from build123d import *

# Parameters (mm, degrees)
ESQUISSE1_R        = 3.9751
BOSS_EXTRU_1_DEPTH = 38.1
BOSS_EXTRU_2_DEPTH = 6.35


with BuildPart() as part:
    # Esquisse1 → Boss.-Extru.1 (new body)
    with BuildSketch(Plane.XY):
        Circle(ESQUISSE1_R)
    extrude(amount=-BOSS_EXTRU_1_DEPTH)

    # Esquisse2 → Boss.-Extru.2 (add)
    with BuildSketch(Plane.XY):
        Polygon((8.248891971, 0), (4.124445986, 7.14375), (-4.124445986, 7.14375), (-8.248891971, 0), (-4.124445986, -7.14375), (4.124445986, -7.14375), align=None)
    extrude(amount=BOSS_EXTRU_2_DEPTH)


solid = part.part
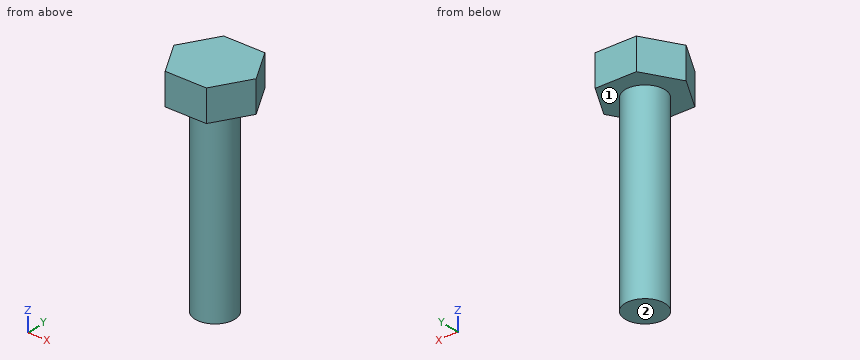
CAD build for the part. Positions are in the model's coordinates, mm. Face numbers are marked on the shaded views. A direction names the side the tool comes from. Coordinates: 2 decimals unless noted, no trailing zeros. Write each loop counter-clockwise with the first axis right and the second up, starting at its lowest first coordinate (ties: lowest second). Pieces come first, ordered by that corner, then holes. Notation, with made-up numbers: M 2.5,6 L 18.5,6 A16 cw 18.5,23 Z; hole C 41,-3 d6. An arc over 180 degrees is marked long. Answer as a JSON object with one key per item and string values. Group by question number.
1) Saw through at A-A (x = 0). Write the cut outline in (y, z).
2) Saw through at B-B (y = 3). Write the cut outline in (x, z), plus the area to 3 significant figures.
3) Pin check, flat tips, straight feed: pin 1 Ø5 at (x, z) = (-3, -3.5) entering from -Y; pin 2 Ø4 at (y, z) = (3.5, -29.5) entering from +X; pin 3 Ø1.5 at (y, z) = (1.5, -25.5) entering from -X. Stop position of each tip, or through.
4) Saw through at C-C (z = -16). Write the cut outline in (x, y), plus the area to 3 significant figures.
5) Saw through at D-D (y = 5.5). Write the cut outline in (x, z).
6) Wall check: line 1 (Z direction, x = 3.75, y = 5.5); line 2 (Y direction, x = -2.5, z = -28); line 3 (Y direction, x = 1, z = -13). Give the ranges that are in metal, low to high. Write a range as from..to.
7) Tool access for the marked faces 1 and 2: list every direction of +Z, -Z, +X, -X, +Y, -Y with a clear straight run to the whole face (end or side of a thin tool).
Values follow:
{
 "1": {"outline": "M -7.14,0 L -3.98,0 L -3.98,-38.1 L 3.98,-38.1 L 3.98,0 L 7.14,0 L 7.14,6.35 L -7.14,6.35 Z"},
 "2": {"outline": "M -6.52,0 L -2.61,0 L -2.61,-38.1 L 2.61,-38.1 L 2.61,0 L 6.52,0 L 6.52,6.35 L -6.52,6.35 Z", "area": "281 mm2"},
 "3": {"pin 1": "stops at y = -3.94", "pin 2": "stops at x = 3.68", "pin 3": "stops at x = -3.9"},
 "4": {"outline": "C 0,0 d7.95", "area": "49.6 mm2"},
 "5": {"outline": "M -5.07,0 L 5.07,0 L 5.07,6.35 L -5.07,6.35 Z"},
 "6": {"line 1": "z = 0..6.35", "line 2": "y = -3.09..3.09", "line 3": "y = -3.85..3.85"},
 "7": {"face 1": "-Z", "face 2": "-Z, +X, -X, +Y, -Y"}
}
